Autodesk Inventor part; units mm, degrees
ref_plane "YZ Plane" through (0, 0, 0) normal (1, 0, 0) x (0, 1, 0)
ref_plane "XZ Plane" through (0, 0, 0) normal (0, 1, 0) x (-1, 0, 0)
ref_plane "XY Plane" through (0, 0, 0) normal (0, 0, 1) x (1, 0, 0)
sketch "スケッチ1" plane through (0, 0, 0) normal (1, 0, 0) x (0, 1, 0)
  line L0 (0, 250) -> (88.1635, -250)
  line L1 (0, 353.3532) -> (0, -370.1192)
  arc A0 (0, 250) -> (88.1635, -250) centre (710.7652, 117.5543) ccw
  arc A1 (0, 250) -> (88.1635, -250) centre (325.1936, 49.5676) ccw
  point P0 (0, 0)
  dimension "d0" = 10
  dimension "d1" = 500
  dimension "d2" = 723
  dimension "d3" = 382
  dimension "d4" = 250
extrude "押し出し1" add sketch "スケッチ1" along normal mid plane 950 contours A0 L1 A1 | A1 L1 A0
fillet "フィレット1" radius 10 1 edges at (0, 0, 250)
fillet "フィレット2" radius 2 1 edges at (0, 88.1635, -250)
shell "シェル1" thickness 1 removed faces 1 at (475, -17.1174, -13.9662)
properties part number "cover_re" material "CFRP"
Check sheet for the modelled part. Datum: model origin and axes. Units: mm. A direction names the side the tool comes from. Round coordinates to 2 decimals unless told otherwise and drop trailing zeros. Loops run counter-clockwise (first coordinate to the right, second up) from the corner with the lowest first, then second, coordinate; pieces in that order, holes last. Notation, with made-up numbers: (-1, -27.75) - (9, -27.75) arc R14 cw to (9, -8.75) - close; hole circle Ø5 at (44.5, -10). An arc over 180 degrees is marked (long way). Answer as CSV lines item,"result". Start each with the question number.
Item 1: Section check A-A (z = -169). Record the boundary of the cut face in (x, y).
Item 2: Release check for a two-part mould opening along Z. For faces 3 (the flat face through (-475, -8, -3)), 4 (the flat face through (-474, -13, -3)), 5 (the cylindrical face through (-6.65, -45.056, -44.451)) record: +Z half, -Z half, draft (parallel to the pull), parting line (faces both ways), or undercut.
Item 3: Depth check by flat-ended pin: P1, Ø8, axis at x = 32.5, y = 15, coming from the -Z side; P2, Ø3, axis at x = 329, y = 44, coming from the +Z side; P3, Ø12, axis at y = -29, z = -117, coming from the -X side; P4, Ø1.5, axis at x = 62, y = 41.5, coming from the -Z side. Enter the tip coordinate at first touch or a pass-through.
Item 4: Scan lines: line 1 (Y direction, x = -322.5, z = -152.5); line 2 (Z direction, x = -312.5, y = 64); line 3 (Y direction, x = 67.5, z = 174). Record each from-to range of solid material in increasing order. Write a range as [from, to].
Item 5: Set-up check for faces 1 (the cylindrical face through (-6.143, 3.054, -35.158)), 2 (the cylindrical face through (-6.65, 4.032, -34.947)): record each of +Z, -Z, +X, -X, +Y, -Y from which the full face is reachable in a straight line by a thin tool's end or side.
Report:
1,outline,"(-475, 11.9) - (475, 11.9) - (475, 13.12) - (-474, 13.12) - (-474, 45.89) - (475, 45.89) - (475, 46.98) - (-475, 46.98) - close"
2,face 3,"draft"
2,face 4,"undercut"
2,face 5,"parting line"
3,P1,"stops at z = -178.84"
3,P2,"stops at z = -158.4"
3,P3,"passes through"
3,P4,"stops at z = -207.08"
4,line 1,"y = [1.01, 2.19], [39.02, 40.09]"
4,line 2,"z = [-229.18, -227.81], [-207.82, -205.59]"
4,line 3,"y = [-35.97, -34.91], [-11.03, -10.03]"
5,face 1,"+X"
5,face 2,"+X, -X, +Y"
